Can you work these out from the model? Positions are in its coordinate system, mm. Give positions to 0.01 mm unless a question says otherwise; leave off trailing zeros. Order: outer loops, then holes, each group sorted by start corner. A loop starts at its lowest first (then second) coordinate and runs counter-clockwise, first axis right, second up. Notation, with made-up numbers: M 31.5,28 L 56.5,28 A23 cw 56.5,43 Z; hole C -13,-17 d4. An arc over 180 degrees is marked long. One line per question, with ' | ' between items. Start each with the question number.
1) If we section it at C-C, the plane z = 12.7: Please give me the cut outline in (x, y), plus the area to 3 significant figures.
2) If we section it at A-A, the plane y = 0: Please give me the cut outline in (x, z), plus the area to 3 significant figures.
3) If we section it at B-B, the plane x = 0: Please give me the cut outline in (y, z).
4) Thinking about a two-plate mould opening in X: for faces 1 (the flat face through (-1, -14, 101.6)), 2 (the cylindrical face through (0.107, -14.875, 61.077)), 3 (the cylindrical face through (-3.62, 16.303, 50.089)), 4 (the cylindrical face through (0.107, -14.875, 10.277)), which applies, +X half, -X half, draft (parallel to the pull), parting line (faces both ways), or undercut?
5) If we section it at D-D, the plane y = -14.5: Please give me the cut outline in (x, z), plus the area to 3 significant figures.
6) Please list where these lines run through material, in increasing order: line 1 along Z through (x, y) = (0, 14.95); line 2 along Y through (x, z) = (0, 58.5); line 3 along Y through (x, z) = (-6.5, 21.5). Write a range as [from, to].
7) I'm going to push flat-ended pins straight in: pin 1 Ø1.5 at (y, z) = (-7, 41) entering from +X; pin 2 Ø4.5 at (x, z) = (0, 12.7) entering from +Y; pin 3 Ø5 at (y, z) = (13, 15.5) entering from -X; pin 4 Ø1 at (x, z) = (5, 19.5) entering from +Y. Where does each tip first touch, or does it pass through?
Autodesk Inventor part; units mm, degrees
ref_plane "Work Plane1" through (0, 0, 0) normal (0, 1, 0) x (0, 0, 1)
ref_plane "XZ Plane" through (0, 0, 0) normal (0, 1, 0) x (-1, 0, 0)
ref_plane "XY Plane" through (0, 0, 0) normal (0, 0, 1) x (1, 0, 0)
sketch "Sketch1" plane through (0, 0, 0) normal (0, 0, 1) x (1, 0, 0)
  circle A0 centre (0, 0) radius 16.7005
  circle A1 centre (0, 0) radius 13.3223
  dimension "d0" = 26.6446
  dimension "d1" = 33.401
extrude "Extrusion1" add sketch "Sketch1" along normal blind 101.6
ref_plane "Work Plane1" through (0, 0, 0) normal (0, 1, 0) x (0, 0, 1)
sketch "Sketch2" plane through (0, 0, 0) normal (0, 1, 0) x (0, 0, 1)
  line L0 (0, -16.7005) -> (101.6, -16.7005)
  line L1 (101.6, 13.3223) -> (101.6, -13.3223)
  line L2 (101.6, 16.7005) -> (101.6, -16.7005)
  line L3 (-20.32, 0) -> (121.92, 0)
  circle A0 centre (63.5, 0) radius 2.4257
  dimension "d5" = 38.1
  dimension "d6" = 4.8514
extrude "Extrusion2" cut sketch "Sketch2" against normal mid plane 1638.3
pattern_linear "Rectangular Pattern1" count 2 spacing 50.8 along (0, 0, -1) of "Extrusion2"
properties part number "FE-00018-02"
Results found:
1) outline: M -2.43,-16.52 L -2.43,-13.1 A13.32 cw -2.43,13.1 L -2.43,16.52 A16.7 ccw Z; M 2.43,-16.52 A16.7 ccw 2.43,16.52 L 2.43,13.1 A13.32 cw 2.43,-13.1 Z | area: 286 mm²
2) outline: M -16.7,0 L -13.32,0 L -13.32,101.6 L -16.7,101.6 Z; M 13.32,0 L 16.7,0 L 16.7,101.6 L 13.32,101.6 Z | area: 686 mm²
3) outline: M -16.7,0 L -13.32,0 L -13.32,10.27 L -16.7,10.27 Z; M -16.7,15.13 L -13.32,15.13 L -13.32,61.07 L -16.7,61.07 Z; M -16.7,65.93 L -13.32,65.93 L -13.32,101.6 L -16.7,101.6 Z; M 13.32,0 L 16.7,0 L 16.7,10.27 L 13.32,10.27 Z; M 13.32,15.13 L 16.7,15.13 L 16.7,61.07 L 13.32,61.07 Z; M 13.32,65.93 L 16.7,65.93 L 16.7,101.6 L 13.32,101.6 Z
4) face 1: draft | face 2: undercut | face 3: parting line | face 4: undercut
5) outline: M -8.29,0 L 8.29,0 L 8.29,101.6 L -8.29,101.6 Z; hole C 0,12.7 d4.85; hole C 0,63.5 d4.85 | area: 1,650 mm²
6) line 1: z = [0, 10.27], [15.13, 61.07], [65.93, 101.6] | line 2: y = [-16.7, -13.32], [13.32, 16.7] | line 3: y = [-15.38, -11.63], [11.63, 15.38]
7) pin 1: stops at x = 15.49 | pin 2: passes through | pin 3: stops at x = -12.99 | pin 4: stops at y = 16.08
